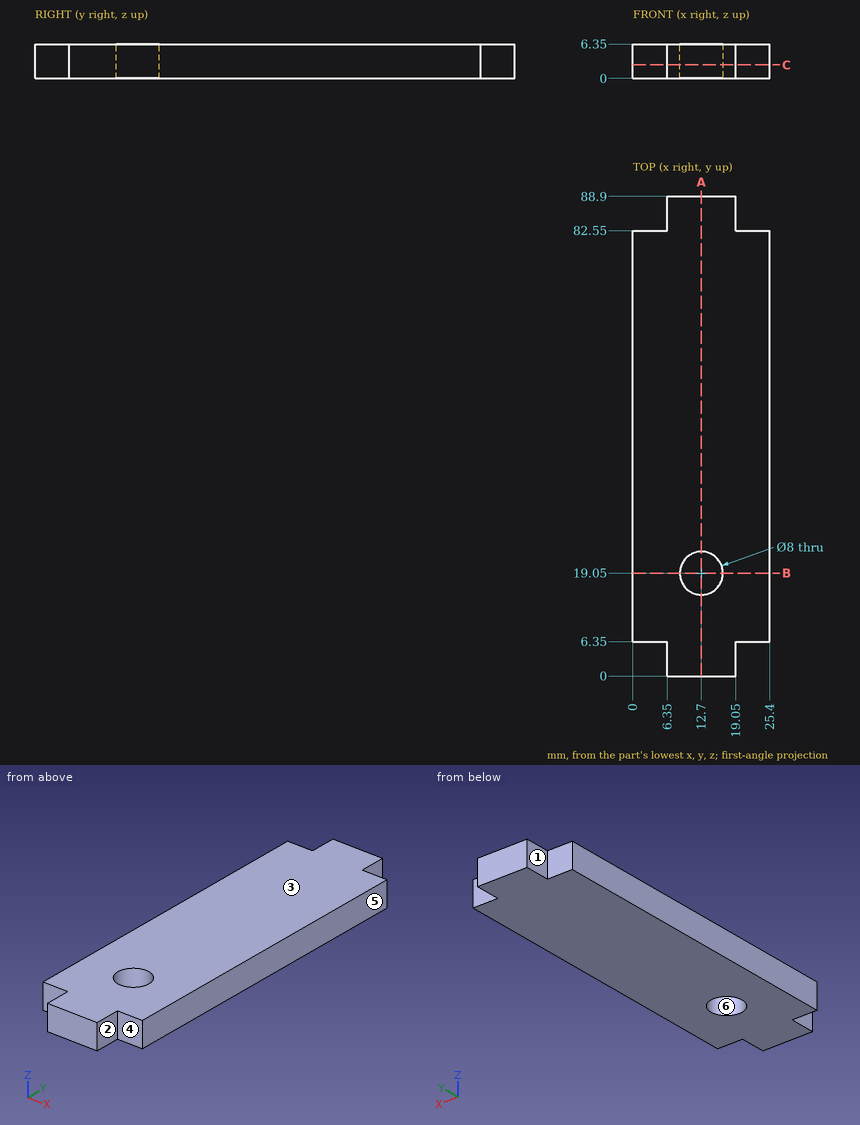
Part print with two shaded views. Sizes in mm from the minimum x, y, z corner. A direction names the side the tool comes from. Coordinates: 2 decimals unless noted, no trailing zeros. Order: outer loops, then holes, each group sorted by start corner. A loop starts at its lowest first (then second) coordinate and runs counter-clockwise, first axis right, second up. Notation, with made-up numbers: M 13.5,26 L 62.5,26 A25 cw 62.5,63 Z; hole C 35.25,-9 d11. An arc over 180 degrees is marked long. One line per question, with ' | ' between items. Start each with the question number.
1. Tool access for the marked faces 1, 2 and 3: list every direction of +Z, -Z, +X, -X, +Y, -Y with a clear straight run to the whole face (end or side of a thin tool).
2. Cut at B-B (y = 19.05). Write the cut outline in (x, z).
3. Mould opens along X. For the marked faces 4, 5 and 6 say: +X half, -X half, draft (parallel to the pull), parting line (faces both ways), or undercut.
4. Flat gauge pins, fed straight in: P1, Ø1.9, axis at y = 84.5, z = 3, coming from the +X side; P2, Ø6.5, axis at x = 12.7, y = 19.05, coming from the -Z side; P3, Ø1.9, axis at x = 22.5, z = 4, coming from the -Y side; P4, Ø1.9, axis at x = 21.5, z = 3.5, coming from the +Y side. Where does each tip first touch, or does it go through?
5. Cut at C-C (z = 2.5). Write the cut outline in (x, y).
6. Cut at A-A (x = 12.7). Write the cut outline in (y, z), plus the area to 3 significant figures.
7. Wall check: line 1 along Y through (x, z) = (12.7, 4.5); line 2 along Y through (x, z) = (15.75, 5.5); line 3 along Y through (x, z) = (2.25, 3.5). Give the ranges that are in metal, low to high. Write a range as [from, to].
The answers:
1) face 1: +Z, -Z, -X, +Y | face 2: +Z, -Z, +X, -Y | face 3: +Z, +X, -X, +Y, -Y
2) outline: M 0,0 L 8.7,0 L 8.7,6.35 L 0,6.35 Z; M 16.7,0 L 25.4,0 L 25.4,6.35 L 16.7,6.35 Z
3) face 4: draft | face 5: +X half | face 6: undercut
4) P1: stops at x = 19.05 | P2: passes through | P3: stops at y = 6.35 | P4: stops at y = 82.55
5) outline: M 0,6.35 L 6.35,6.35 L 6.35,0 L 19.05,0 L 19.05,6.35 L 25.4,6.35 L 25.4,82.55 L 19.05,82.55 L 19.05,88.9 L 6.35,88.9 L 6.35,82.55 L 0,82.55 Z; hole C 12.7,19.05 d8
6) outline: M 0,0 L 15.05,0 L 15.05,6.35 L 0,6.35 Z; M 23.05,0 L 88.9,0 L 88.9,6.35 L 23.05,6.35 Z | area: 514 mm2
7) line 1: y = [0, 15.05], [23.05, 88.9] | line 2: y = [0, 16.46], [21.64, 88.9] | line 3: y = [6.35, 82.55]
